from build123d import *

# Parameters (mm, degrees)
F0_W     = 63.5
F0_H     = 38.1
F1_DEPTH = 25.4
F3_DEPTH = 25.4


with BuildPart() as f1:
    # F0 (on Front) → F1 (new body)
    with BuildSketch(Plane.XZ):
        with Locations((31.75, 19.05)):
            Rectangle(F0_W, F0_H)
    extrude(amount=F1_DEPTH)

    # F2 (on face) → F3 (cut)
    with BuildSketch(Plane.XZ.offset(25.4)):
        with BuildLine():
            ThreePointArc((13.789488, 38.1), (28.528607, 12.974347), (50.8, 31.75))
            ThreePointArc((50.8, 31.75), (50.525653, 34.971393), (49.710512, 38.1))
            Line((49.710512, 38.1), (13.789488, 38.1))
        make_face()
    extrude(amount=-F3_DEPTH, mode=Mode.SUBTRACT)


solid = f1.part
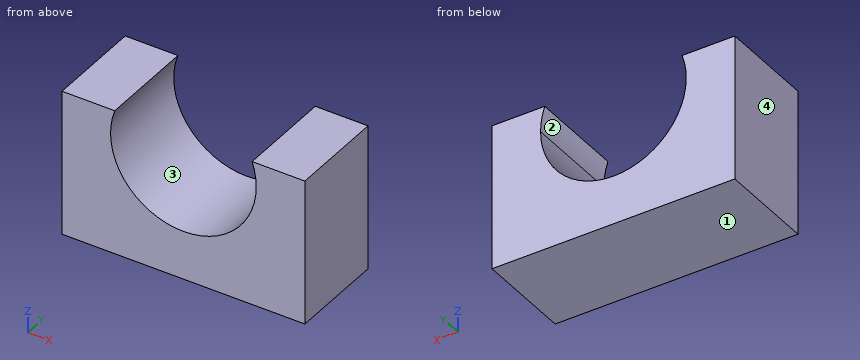
CAD build for the part. Positions are in the model's coordinates, mm. Face numbers are marked on the shaded views. Coordinates: 2 decimals unless noted, no trailing zeros. Loops run counter-clockwise (first coordinate to the right, second up) from the corner with the lowest first, then second, coordinate; pieces in that order, holes last. Notation, with made-up numbers: (32, -4.5) - (58, -4.5) arc R30 ccw to (58, 24.5) - close; hole circle Ø9 at (4, -28). An arc over 180 degrees is marked (long way). Write item = value, one per line. Start each with the question number.
Q1. Drill centre lines: L1, parallel to X at y = -13.5, z = 31.75; L2, parallel to X at y = -17.75, z = 19.5; L3, parallel to Z at x = 31.75, y = -15. Where is each one in solid material? Low to high.
Q2. Cut at D-D, the plane x = 31.75. List the corners of the cut face in (y, z).
Q3. Flat gauge pins, fed straight in: pin 1 Ø1 at (y, z) = (-14, 25.5) entering from -X; pin 2 Ø1 at (x, y) = (41.5, -15.5) entering from +Z; pin 3 Ø1.5 at (x, y) = (20.5, -10) entering from +Z. Where does each tip first touch, or does it go through?
Q4. Cut at C-C, the plane x = 22.5. List the corners of the cut face in (y, z).
Q5. Cut at A-A, the plane z = 13.5. List the corners of the cut face in (x, y).
Q6. Pull direction Z, two halves, no side cores. Call the marked faces 1, 2, 3 and 4: pulls with the +Z half, pulls with the -Z half, needs draft (parallel to the pull), parting line crosses it, or undercut.
Q7. Cut at B-B, the plane y = -17. List the corners of the cut face in (x, z).
Computed:
q1.L1 = 0 to 12.7, 50.8 to 63.5
q1.L2 = 0 to 17.16, 46.34 to 63.5
q1.L3 = 0 to 12.7
q2.outline = (-25.4, 0) - (0, 0) - (0, 12.7) - (-25.4, 12.7) - close
q3.pin_1 = 0
q3.pin_2 = 15.69
q3.pin_3 = 16.95
q4.outline = (-25.4, 0) - (0, 0) - (0, 15.1) - (-25.4, 15.1) - close
q5.outline = (0, -25.4) - (26.29, -25.4) - (26.29, 0) - (0, 0) - close; (37.21, -25.4) - (63.5, -25.4) - (63.5, 0) - (37.21, 0) - close
q6.face_1 = pulls with the -Z half
q6.face_2 = undercut
q6.face_3 = undercut
q6.face_4 = needs draft
q7.outline = (0, 0) - (63.5, 0) - (63.5, 38.1) - (49.71, 38.1) arc R19.05 cw to (50.8, 31.75) arc R19.05 cw (long way) to (13.79, 38.1) - (0, 38.1) - close
